```python
from build123d import *

# Parameters (mm, degrees)
SKETCH11_W          = 38.1
SKETCH11_H          = 53.975
SKETCH11_R          = 1.651
SKETCH11_R_2        = 1.5875
SKETCH11_R_3        = 1.27
BOSS_EXTRUDE1_DEPTH = 3.175
SKETCH12_W          = 44.45
SKETCH12_H          = 60.325
SKETCH12_W_2        = 38.1
SKETCH12_H_2        = 53.975
BOSS_EXTRUDE2_DEPTH = 6.35
SKETCH13_W          = 6.858
SKETCH13_H          = 10.16
SKETCH13_R          = 1.651
SKETCH13_W_2        = 10.16
SKETCH13_H_2        = 6.858
BOSS_EXTRUDE3_DEPTH = 6.35
SKETCH14_R          = 3.6195
SKETCH14_R_2        = 1.5875
SKETCH14_R_3        = 3.302
SKETCH14_R_4        = 1.27
BOSS_EXTRUDE4_DEPTH = 10.16
FILLET2_R           = 1.27


with BuildPart() as part:
    # Sketch11 → Boss-Extrude1 (new body)
    with BuildSketch(Plane(origin=(0, 0, 0), x_dir=(0, 0, -1), z_dir=(1, 0, 0))):
        with Locations((0, 9.2075)):
            Rectangle(SKETCH11_W, SKETCH11_H)
        with Locations((0, 16.256)):
            Circle(SKETCH11_R, mode=Mode.SUBTRACT)
        with Locations((6.7945, 0)):
            Circle(SKETCH11_R_2, mode=Mode.SUBTRACT)
        with Locations((10.336274795, -10.336274795)):
            Circle(SKETCH11_R_3, mode=Mode.SUBTRACT)
        with Locations(Location((-10.336274795, -10.336274795, 0), (0, 0, 180))):
            Circle(SKETCH11_R_3, mode=Mode.SUBTRACT)
        with Locations(Location((-6.7945, 0, 0), (0, 0, 180))):
            Circle(SKETCH11_R_2, mode=Mode.SUBTRACT)
    extrude(amount=-BOSS_EXTRUDE1_DEPTH)

    # Sketch12 → Boss-Extrude2 (add)
    with BuildSketch(Plane(origin=(0, 0, 0), x_dir=(0, 0, -1), z_dir=(1, 0, 0))):
        with Locations((0, 9.2075)):
            Rectangle(SKETCH12_W, SKETCH12_H)
        with Locations((0, 9.2075)):
            Rectangle(SKETCH12_W_2, SKETCH12_H_2, mode=Mode.SUBTRACT)
    extrude(amount=-BOSS_EXTRUDE2_DEPTH)

    # Sketch13 → Boss-Extrude3 (add)
    # profile 1 of 3: a face of its own
    with BuildSketch(Plane(origin=(0, 0, 0), x_dir=(0, 0, -1), z_dir=(1, 0, 0))):
        with Locations((-25.654, -12.7)):
            Rectangle(SKETCH13_W, SKETCH13_H)
        with Locations((-25.654, -12.7)):
            Circle(SKETCH13_R, mode=Mode.SUBTRACT)
    # profile 2 of 3: a face of its own
    with BuildSketch(Plane(origin=(0, 0, 0), x_dir=(0, 0, -1), z_dir=(1, 0, 0))):
        with Locations((0, 42.799)):
            Rectangle(SKETCH13_W_2, SKETCH13_H_2)
        with Locations((0, 42.799)):
            Circle(SKETCH13_R, mode=Mode.SUBTRACT)
    # profile 3 of 3: a face of its own
    with BuildSketch(Plane(origin=(0, 0, 0), x_dir=(0, 0, -1), z_dir=(1, 0, 0))):
        with Locations((25.654, -12.7)):
            Rectangle(SKETCH13_W, SKETCH13_H)
        with Locations((25.654, -12.7)):
            Circle(SKETCH13_R, mode=Mode.SUBTRACT)
    extrude(amount=-BOSS_EXTRUDE3_DEPTH)

    # Sketch14 → Boss-Extrude4 (add)
    # profile 1 of 4: a face of its own
    with BuildSketch(Plane.ZY.offset(3.175)):
        with Locations(Location((-6.7945, 0, 0), (0, 0, 180))):
            Circle(SKETCH14_R)
        with Locations(Location((-6.7945, 0, 0), (0, 0, 180))):
            Circle(SKETCH14_R_2, mode=Mode.SUBTRACT)
    # profile 2 of 4: a face of its own
    with BuildSketch(Plane.ZY.offset(3.175)):
        with Locations(Location((6.7945, 0, 0), (0, 0, 180))):
            Circle(SKETCH14_R)
        with Locations((6.7945, 0)):
            Circle(SKETCH14_R_2, mode=Mode.SUBTRACT)
    # profile 3 of 4: a face of its own
    with BuildSketch(Plane.ZY.offset(3.175)):
        with Locations(Location((-10.336274795, -10.336274795, 0), (0, 0, 180))):
            Circle(SKETCH14_R_3)
        with Locations(Location((-10.336274795, -10.336274795, 0), (0, 0, 180))):
            Circle(SKETCH14_R_4, mode=Mode.SUBTRACT)
    # profile 4 of 4: a face of its own
    with BuildSketch(Plane.ZY.offset(3.175)):
        with Locations(Location((10.336274795, -10.336274795, 0), (0, 0, 180))):
            Circle(SKETCH14_R_3)
        with Locations((10.336274795, -10.336274795)):
            Circle(SKETCH14_R_4, mode=Mode.SUBTRACT)
    extrude(amount=BOSS_EXTRUDE4_DEPTH)

    # Fillet2
    fillet2_edges = [part.edges().sort_by_distance(p)[0] for p in [
        (-3.175, 39.37, 22.225),
        (-3.175, 39.37, -22.225),
        (-3.175, -20.955, -22.225),
        (-3.175, -20.955, 22.225),
        (-3.175, -7.62, 29.083),
        (-3.175, -17.78, 29.083),
        (-3.175, -17.78, 22.225),
        (-3.175, -7.62, 22.225),
        (-3.175, 46.228, 5.08),
        (-3.175, 39.37, 5.08),
        (-3.175, 39.37, -5.08),
        (-3.175, 46.228, -5.08),
        (-3.175, -17.78, -29.083),
        (-3.175, -7.62, -29.083),
        (-3.175, -7.62, -22.225),
        (-3.175, -17.78, -22.225),
    ]]
    fillet(fillet2_edges, radius=FILLET2_R)


solid = part.part
```
Check sheet for the modelled part. Datum: model origin and axes. Units: mm. A direction names the side the tool comes from. Give positions to 0.01 mm unless a question says otherwise; leave off trailing zeros. Write each loop counter-clockwise with the first axis right and the second up, starting at its lowest first coordinate (ties: lowest second). Pieces come first, ordered by that corner, then holes. Notation, with made-up numbers: (-5.75, -16.5) - (50.25, -16.5) arc R22 ccw to (50.25, 18.5) - close; hole circle Ø3 at (55, -6.75). An arc over 180 degrees is marked (long way). Answer as a JSON object with one key per item and string values. Group by question number.
1) Sectioned sample at B-B (z = 0). Record the cut outline in (x, y) (3 decimals).
2) Thickness scan on probe 1 along Y at (x, z) = (-4.5, 0) (3 decimals); probe 2 along Z at (x, y) = (-4.75, 32) (3 decimals); probe 3 along X at (y, z) = (6.5, -17) (3 decimals). Record the ranges inside material, lowest first. Write a range as from..to.
3) Sectioned sample at C-C (z = 26). Record the cut outline in (x, y).
4) Release check for a two-part mould opening along Z. For faces 5 (the face through (-5, -17.78, 0)), 6 (the face through (-13.335, 0.8, -8.4)), 7 (the face through (-3, -13, -29.083)) record: pulls with the +Z half, pulls with the -Z half, needs draft (parallel to the pull), parting line crosses it, or undercut.
5) Sectioned sample at D-D (y = -15.5). Record the cut outline in (x, z) (3 decimals), then the cut area to 3 significant figures.
6) Depth check by flat-ended pin: P1, Ø4, axis at y = 31, z = 14, coming from the +X side; P2, Ø1.6, axis at x = -5, z = -8, coming from the +Y side; P3, Ø1.3, axis at x = -3, z = 26.5, coming from the +Y side; P4, Ø5, axis at y = 8, z = -0.5, coming from the -X side (3 decimals). Enter the tip coordinate at first touch or a pass-through.
7) Access from +Z, -Z, +X, -X, +Y, -Y to the whole of each face (thin tool, end or side, straight path). Record for faces 1 (the face through (-5, 9, 19.05)), 2 (the face through (-3, -7.62, 26)), 3 (the face through (-3, 39.37, -14)), 4 (the face through (-3, -17.78, -26)).
8) Sectioned sample at A-A (y = 0). Record the cut outline in (x, z) (3 decimals), then the cut area to 3 significant figures.
Geometry results:
{
 "1": {"outline": "(-6.35, -20.955) - (0, -20.955) - (0, 14.605) - (-3.175, 14.605) - (-3.175, -17.78) - (-6.35, -17.78) - close; (-6.35, 36.195) - (-3.175, 36.195) - (-3.175, 17.907) - (0, 17.907) - (0, 41.148) - (-6.35, 41.148) - close; (-6.35, 44.45) - (0, 44.45) - (0, 46.228) - (-6.35, 46.228) - close"},
 "2": {"probe 1": "y = -20.955..-17.78, 36.195..41.148, 44.45..46.228", "probe 2": "z = -22.225..-19.05, 19.05..22.225", "probe 3": "x = -3.175..0"},
 "3": {"outline": "(-6.35, -17.78) - (0, -17.78) - (0, -14.31) - (-6.35, -14.31) - close; (-6.35, -11.09) - (0, -11.09) - (0, -7.62) - (-6.35, -7.62) - close"},
 "4": {"face 5": "undercut", "face 6": "needs draft", "face 7": "pulls with the -Z half"},
 "5": {"outline": "(-6.35, -29.083) - (0, -29.083) - (0, 29.083) - (-6.35, 29.083) - (-6.35, 19.05) - (-3.175, 19.05) - (-3.175, -19.05) - (-6.35, -19.05) - close", "area": "248 mm^2"},
 "6": {"P1": "stops at x = 0", "P2": "stops at y = 39.37", "P3": "stops at y = -7.62", "P4": "stops at x = -3.175"},
 "7": {"face 1": "-X", "face 2": "+Z, +X, -X, +Y", "face 3": "-Z, +X, -X, +Y", "face 4": "-Z, +X, -X, -Y"},
 "8": {"outline": "(-13.335, -10.414) - (-3.175, -10.414) - (-3.175, -19.05) - (-6.35, -19.05) - (-6.35, -22.225) - (0, -22.225) - (0, -8.382) - (-13.335, -8.382) - close; (-13.335, -5.207) - (0, -5.207) - (0, 5.207) - (-13.335, 5.207) - (-13.335, 3.175) - (-3.175, 3.175) - (-3.175, -3.175) - (-13.335, -3.175) - close; (-13.335, 8.382) - (0, 8.382) - (0, 22.225) - (-6.35, 22.225) - (-6.35, 19.05) - (-3.175, 19.05) - (-3.175, 10.414) - (-13.335, 10.414) - close", "area": "224 mm^2"}
}
